Can you work these out from the model? Positions are in its coordinate system, mm. A direction names the side the tool comes from. Coordinates: 2 decimals unless noted, no trailing zeros. Order: outer loops, then holes, each group sorted by start corner. A loop starts at its lowest first (then second) coordinate and runs counter-clockwise, first axis right, second up. Notation, with made-up numbers: (51, 22) -> (99, 22) arc R19 cw to (99, 58) -> close; hole circle Ø8 at (59.5, -29). An arc over 180 degrees is marked (long way). Write item = value, one per line.
Autodesk Inventor part; units mm, degrees
ref_plane "Arbeitsebene3" through (-3.4226, 4.8, -13.6708) normal (0.2249, 0.9744, -0.004) x (0.0178, 0, 0.9998)
ref_plane "YZ Plane" through (0, 0, 0) normal (1, 0, 0) x (0, 1, 0)
ref_plane "XZ Plane" through (0, 0, 0) normal (0, 1, 0) x (-1, 0, 0)
sketch "Skizze1" plane through (0, 0, 0) normal (0, 1, 0) x (-1, 0, 0)
  line L0 (0, 0) -> (21.4435, 0) construction
  line L1 (21.4435, 0) -> (21.4435, -17.7713) construction
  line L2 (21.4435, -17.7713) -> (0, -17.7713) construction
  line L3 (0, -17.7713) -> (0, 0) construction
  arc A0 (3.4429, -6.1124) -> (3.5369, -12.2987) centre (13.9264, -9.047) ccw
  arc A1 (3.5369, -12.2987) -> (17.7561, -12.2571) centre (10.6298, -6.5721) ccw
  arc A2 (17.8481, -6.152) -> (3.4429, -6.1124) centre (10.6298, -11.844) ccw
  arc A3 (17.7561, -12.2571) -> (17.8481, -6.152) centre (7.348, -9.047) ccw
  line L4 (3.0399, -9.047) -> (18.2399, -9.047)
  line L5 (10.6298, -2.6515) -> (10.6298, -15.6882)
  dimension "d9" = 15.2
  dimension "d12" = 13.0368
sketch "Skizze2" plane through (0, 0, 0) normal (0, 1, 0) x (-1, 0, 0)
  line L0 (0, 0) -> (21.0912, 0) construction
  line L1 (21.0912, 0) -> (21.0912, -24.0698) construction
  line L2 (21.0912, -24.0698) -> (0, -24.0698) construction
  line L3 (0, -24.0698) -> (0, 0) construction
  line L4 (17.3479, -12.3442) -> (17.5564, -17.8355)
  line L5 (0, -15.4153) -> (21.0912, -15.022)
  point P0 (17.4522, -15.0899)
  point P1 (17.8576, -15.0823)
  point P2 (2.6602, -15.3657)
  point P3 (10.1167, -10.9016)
  point P4 (10.0352, -15.2282)
  point P5 (10.3203, -19.614)
  point P6 (15.9484, -15.1179)
  point P7 (4.4034, -15.3332)
  dimension "d38" = 15.2
  dimension "d47" = 8.7147
sketch "Skizze3" plane through (0, 0, 0) normal (0, 1, 0) x (-1, 0, 0)
  line L0 (0, 0) -> (41.0457, 0) construction
  line L1 (41.0457, 0) -> (41.0457, -50.0176) construction
  line L2 (41.0457, -50.0176) -> (0, -50.0176) construction
  line L3 (0, -50.0176) -> (0, 0) construction
  arc A0 (26.8609, -29.1094) -> (14.9484, -29.1094) centre (20.9046, -43.0907) ccw
  arc A1 (14.9484, -37.9624) -> (26.8609, -37.9624) centre (20.9046, -23.981) ccw
  line L4 (26.8609, -29.1094) -> (26.8609, -37.9624)
  line L5 (14.9484, -37.9624) -> (14.9484, -29.1094)
  point P0 (20.7813, -28.8717)
  point P1 (20.996, -37.5841)
  dimension "d49" = 8.715
  dimension "d57" = 15.1972
  dimension "d58" = 15.1972
  dimension "d59" = 11.9125
  dimension "d67" = 8.853
  dimension "d69" = 0
  dimension "d70" = 8.853
sketch "Skizze4" plane through (0, 0, 0) normal (0, 1, 0) x (-1, 0, 0)
  arc A0 (19.2206, -6.6251) -> (3.7078, -6.5825) centre (11.4473, -12.755) ccw
  arc A1 (19.1216, -13.1996) -> (19.2206, -6.6251) centre (7.9131, -9.7427) ccw
  arc A2 (3.8091, -13.2445) -> (19.1216, -13.1996) centre (11.4473, -7.0776) ccw
  arc A3 (3.7078, -6.5825) -> (3.8091, -13.2445) centre (14.9974, -9.7427) ccw
  arc A4 (20.1996, -6.1308) -> (2.731, -6.0835) centre (11.4473, -12.755) ccw
  arc A5 (20.0894, -13.7103) -> (20.1996, -6.1308) centre (7.9131, -9.7427) ccw
  arc A6 (2.8436, -13.7601) -> (20.0894, -13.7103) centre (11.4473, -7.0776) ccw
  arc A7 (2.731, -6.0835) -> (2.8436, -13.7601) centre (14.9974, -9.7427) ccw
  point P0 (0, 0)
  dimension "d60" = 1.077
extrude "Extrusion1" add sketch "Skizze4" along normal blind 3.1
sketch "Skizze8" plane through (0, 3.1, 0) normal (0, 1, 0) x (1, 0, 0)
  line L0 (-17.4719, 5.508) -> (-17.4719, 14.361)
  arc A0 (-17.4719, 5.508) -> (-5.5595, 5.508) centre (-11.5157, 19.4893) ccw
  arc A1 (-5.5595, 14.361) -> (-17.4719, 14.361) centre (-11.5157, 0.3796) ccw
  line L1 (-5.5595, 14.361) -> (-5.5595, 5.508)
  line L2 (-17.4719, 5.508) -> (-5.5595, 14.361) construction
  line L3 (-17.4719, 14.361) -> (-5.5595, 5.508) construction
  arc A2 (-19.1216, 13.1996) -> (-19.2206, 6.6251) centre (-7.9131, 9.7427) ccw construction
  arc A3 (-3.8091, 13.2445) -> (-19.1216, 13.1996) centre (-11.4473, 7.0776) ccw construction
  arc A4 (-3.7078, 6.5825) -> (-3.8091, 13.2445) centre (-14.9974, 9.7427) ccw construction
  arc A5 (-19.2206, 6.6251) -> (-3.7078, 6.5825) centre (-11.4473, 12.755) ccw construction
  arc A6 (-20.1996, 6.1308) -> (-2.731, 6.0835) centre (-11.4473, 12.755) ccw
  arc A7 (-2.731, 6.0835) -> (-2.8436, 13.7601) centre (-14.9974, 9.7427) ccw
  arc A8 (-2.8436, 13.7601) -> (-20.0894, 13.7103) centre (-11.4473, 7.0776) ccw
  arc A9 (-20.0894, 13.7103) -> (-20.1996, 6.1308) centre (-7.9131, 9.7427) ccw
  line L4 (-19.2206, 6.6251) -> (-3.8091, 13.2445) construction
  line L5 (-19.1216, 13.1996) -> (-3.7078, 6.5825) construction
  point P0 (0, 0)
  point P1 (-11.5157, 9.9345)
  point P2 (-11.5157, 9.9345)
extrude "Extrusion3" add sketch "Skizze8" along normal blind 0.5
sketch "Skizze9" plane through (0, 0, 0) normal (0, 0, 1) x (1, 0, 0)
  line L0 (-2.731, 0) -> (-20.1996, 0) construction
  line L1 (-2.731, 0) -> (-2.731, 3.6) construction
  line L2 (-20.1996, 3.6) -> (-2.731, 3.6) construction
  line L3 (-20.1996, 0) -> (-20.1996, 3.6) construction
  line L4 (-3.8091, 0) -> (-19.1216, 0)
  line L5 (-11.4653, 0) -> (-12.0653, 0)
  line L6 (-12.0653, 0) -> (-12.0653, 1.55)
  arc A0 (-11.4653, 2.15) -> (-12.0653, 1.55) centre (-11.4653, 1.55) ccw
  line L7 (-11.4653, 1.55) -> (-11.4653, 2.15) construction
  line L8 (-11.4653, 1.55) -> (-12.0653, 1.55) construction
  line L9 (-11.4653, 0) -> (-11.4653, 6.3928) construction
  line L10 (-20.1996, 0) -> (-2.731, 0) construction
  line L11 (-10.8653, 0) -> (-10.8653, 1.55)
  arc A1 (-10.8653, 1.55) -> (-11.4653, 2.15) centre (-11.4653, 1.55) ccw
  line L12 (-11.4653, 0) -> (-10.8653, 0)
  point P0 (0, 0)
  dimension "d75" = 0.6
  dimension "d76" = 90
  dimension "d77" = 1.55
extrude "Extrusion4" cut sketch "Skizze9" against normal up to next
sketch "Skizze10" plane through (0, 0, 0) normal (0, 1, 0) x (-1, 0, 0)
  arc A0 (5.5595, -14.361) -> (17.4719, -14.361) centre (11.5157, -0.3796) ccw
  line L0 (5.5595, -14.361) -> (5.5595, -5.508)
  arc A1 (17.4719, -5.508) -> (5.5595, -5.508) centre (11.5157, -19.4893) ccw
  line L1 (17.4719, -5.508) -> (17.4719, -14.361)
  arc A2 (20.1996, -6.1308) -> (2.731, -6.0835) centre (11.4473, -12.755) ccw
  arc A3 (2.731, -6.0835) -> (2.8436, -13.7601) centre (14.9974, -9.7427) ccw
  arc A4 (2.8436, -13.7601) -> (20.0894, -13.7103) centre (11.4473, -7.0776) ccw
  arc A5 (20.0894, -13.7103) -> (20.1996, -6.1308) centre (7.9131, -9.7427) ccw
  arc A6 (20.1996, -6.1308) -> (2.731, -6.0835) centre (11.4473, -12.755) ccw
  line L2 (5.5595, -14.361) -> (5.5595, -5.508) construction
  line L3 (5.5595, -9.9345) -> (-7.2798, -9.9345) construction
  line L4 (3.7452, -4.9345) -> (-3.2387, -5.9345)
  line L5 (-3.2387, -5.9345) -> (-3.2387, -9.9345)
  line L6 (3.9282, -14.9607) -> (-3.2387, -13.9345)
  line L7 (-3.2387, -13.9345) -> (-3.2387, -9.9345)
  line L8 (17.4719, -5.508) -> (17.4719, -14.361) construction
  line L9 (17.4719, -9.9345) -> (23.9782, -9.9345) construction
  line L10 (22.5662, -4.9345) -> (14.2748, -4.9345) construction
  arc A7 (2.731, -6.0835) -> (2.8436, -13.7601) centre (14.9974, -9.7427) ccw construction
  line L11 (26.2701, -9.9345) -> (26.2701, -5.9345)
  line L12 (26.2701, -5.9345) -> (19.1494, -4.9345)
  line L13 (26.2701, -9.9345) -> (26.2701, -13.9345)
  line L14 (26.2701, -13.9345) -> (18.967, -14.9601)
  point P0 (0, 0)
  point P1 (3.7452, -14.9345)
  point P2 (2.1983, -9.9345)
  point P3 (2.1983, -9.9345)
  point P4 (19.1494, -14.9345)
  dimension "d80" = 5
  dimension "d81" = 5
  dimension "d82" = 8.7982
  dimension "d83" = 8.7982
  dimension "d84" = 4
  dimension "d85" = 4
extrude "Extrusion5" add sketch "Skizze10" along normal up to surface (3.6 mm away) contours A2 L12 L11 L13 L14 A4 A5 | A2 A3 A4 L6 L7 L5 L4
sketch "Skizze13" plane through (0, 0, 0) normal (0, -1, 0) x (1, 0, 0)
  line L0 (-3.7452, -4.9345) -> (3.2387, -5.9345)
  line L1 (3.2387, -13.9345) -> (-3.9282, -14.9607)
  arc A0 (-3.8091, -13.2445) -> (-3.7078, -6.5825) centre (-14.9974, -9.7427) ccw
  arc A1 (-3.3813, -14.9345) -> (-2.5876, -6.9345) centre (-14.9974, -9.7427) ccw
  line L2 (3.2387, -5.9345) -> (3.2387, -13.9345)
  line L3 (3.2387, -6.9345) -> (-2.5876, -6.9345)
  line L4 (3.2387, -14.9345) -> (-3.3813, -14.9345)
  point P0 (0, 0)
  dimension "d92" = 1
  dimension "d104" = 1
  dimension "d105" = 1
sketch "Skizze12" plane through (0, 0, 0) normal (0, -1, 0) x (1, 0, 0)
  arc A0 (-3.5369, -12.2987) -> (-3.4429, -6.1124) centre (-13.9264, -9.047) ccw
  arc A1 (-17.7561, -12.2571) -> (-3.5369, -12.2987) centre (-10.6298, -6.5721) ccw
  arc A2 (-17.8481, -6.152) -> (-17.7561, -12.2571) centre (-7.348, -9.047) ccw
  arc A3 (-11.2465, -2.6722) -> (-17.8481, -6.152) centre (-10.6298, -11.844) ccw
  line L0 (-11.2465, -2.6722) -> (-11.2465, -1.6701)
  arc A4 (-11.2465, -1.6701) -> (-17.9952, -4.7985) centre (-10.6298, -11.844) ccw
  line L1 (-25.4478, -5.693) -> (-17.9952, -4.7985)
  line L2 (-25.4478, -12.757) -> (-25.4478, -5.693)
  line L3 (-17.8374, -13.6705) -> (-25.4478, -12.757)
  arc A5 (-17.8374, -13.6705) -> (-3.4226, -13.6708) centre (-10.6298, -6.5721) ccw
  line L4 (-17.9952, -4.7985) -> (-17.963, -6.6068)
  line L5 (-17.8695, -11.8632) -> (-17.8374, -13.6705)
  arc A6 (-2.3529, -11.757) -> (-2.2753, -6.693) centre (-13.9264, -9.047) ccw
  line L6 (4.0611, -5.693) -> (4.0611, -6.693)
  line L7 (-3.2644, -4.7985) -> (4.0611, -5.693)
  arc A7 (-3.2644, -4.7985) -> (-10.0465, -1.6682) centre (-10.6298, -11.844) ccw
  line L8 (-10.0465, -1.6682) -> (-10.0465, -2.67)
  arc A8 (-3.4429, -6.1124) -> (-10.0465, -2.67) centre (-10.6298, -11.844) ccw
  line L9 (4.0611, -12.757) -> (-3.4226, -13.6708)
  line L10 (4.0611, -11.757) -> (4.0611, -12.757)
  line L11 (4.0611, -11.757) -> (-2.3529, -11.757)
  line L12 (-2.2753, -6.693) -> (4.0611, -6.693)
  point P0 (0, 0)
properties part number "Main"
Item 1: I'm going to push a flat-ended pin straight in: P1, Ø2, axis at x = -20.5, y = 2, coming from the -Z side. Where does the tip first touch, or does it pass through?
A:
P1 = -14.89
Item 2: I want a section at B-B, the plane y = 2.5. Please give me the cut outline in (x, z) (1 decimal), plus the area to 3 significant figures.
A:
outline = (-26.3, -13.9) -> (-19, -15) arc R10.9 ccw to (-3.9, -15) -> (3.2, -13.9) -> (3.2, -5.9) -> (-3.7, -4.9) arc R11 ccw to (-19.1, -4.9) -> (-26.3, -5.9) -> close; hole (-19.2, -6.6) arc R11.7 ccw to (-19.1, -13.2) arc R9.8 ccw to (-3.8, -13.2) arc R11.7 ccw to (-3.7, -6.6) arc R9.9 ccw to start
area = 160 mm2
Item 3: I want a section at C-C, the plane y = 1.25. Please give me the cut outline in (x, z) (1 decimal), plus the area to 3 significant figures.
A:
outline = (-26.3, -13.9) -> (-19, -15) arc R10.9 ccw to (-3.9, -15) -> (3.2, -13.9) -> (3.2, -5.9) -> (-3.7, -4.9) arc R11 ccw to (-10.9, -1.8) -> (-10.9, -2.9) arc R9.9 cw to (-3.7, -6.6) arc R11.7 cw to (-3.8, -13.2) arc R9.8 cw to (-19.1, -13.2) arc R11.7 cw to (-19.2, -6.6) arc R9.9 cw to (-12.1, -2.9) -> (-12.1, -1.8) arc R11 ccw to (-19.1, -4.9) -> (-26.3, -5.9) -> close
area = 159 mm2
Item 4: If we mould it in two halves opening along X, with no side actions, what happens to faces 6 (the cylindrical face through (-11.56, 1.77, -17.97)), 7 (the cylindrical face through (-11.35, 2.562, -2.856)), 8 (the flat face through (-9, 0, -17)), 9 (the flat face through (-22.67, 1.77, -14.44))? For each: pulls with the +X half, pulls with the -X half, needs draft (parallel to the pull), parting line crosses it, or undercut.
A:
face_6 = parting line crosses it
face_7 = undercut
face_8 = needs draft
face_9 = pulls with the -X half
Item 5: If I drill on probe 1 along X at (y, z) = (2.6, -9.75); probe 2 along X at (y, z) = (3.35, -8.75); probe 3 along Y at (x, z) = (-9.25, -3.25), over which ranges is the centre line in solid material (lowest first)?
A:
probe_1 = -26.27 to -19.64, -3.27 to 3.24
probe_2 = -26.27 to -17.47, -5.56 to 3.24
probe_3 = 3.1 to 3.6
Item 6: I want a section at D-D, the plane x = -2. Please give me the cut outline in (y, z), plus the area to 3 significant figures.
A:
outline = (0, -14.68) -> (3.6, -14.68) -> (3.6, -5.18) -> (0, -5.18) -> close
area = 34.2 mm2
Item 7: For faces 1 (the cylindrical face through (-11.43, 3.347, -4.292)), 2 (the cylindrical face through (-11.45, 2.15, -2.32)), 3 (the flat face through (-11, 3.1, -4)), 4 (the flat face through (3.239, 2, -10)), 5 (the cylindrical face through (-11.33, 2.57, -1.78)), which set-ups out of +Z, -Z, +X, -X, +Y, -Y let a thin tool reach every point of the face, with its end or its side?
A:
face_1 = +Y, -Y
face_2 = +Z, -Y
face_3 = -Y
face_4 = +Z, -Z, +X, +Y, -Y
face_5 = +Z, +Y, -Y
Item 8: I want a section at A-A, the plane x = -14.5. Please give me the cut outline in (y, z), plus the area to 3 significant figures.
A:
outline = (0, -17.54) -> (3.6, -17.54) -> (3.6, -15.28) -> (3.1, -15.28) -> (3.1, -16.41) -> (0, -16.41) -> close; (0, -3.34) -> (3.1, -3.34) -> (3.1, -4.59) -> (3.6, -4.59) -> (3.6, -2.21) -> (0, -2.21) -> close
area = 9.30 mm2
